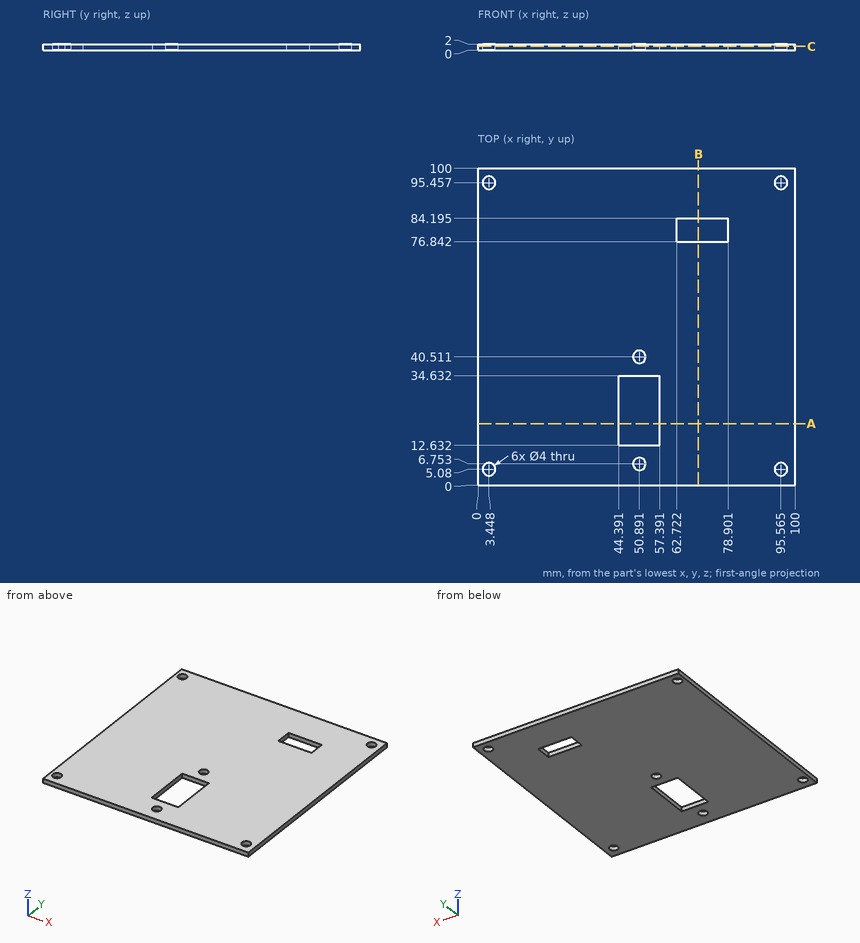
Input: dimensioned drawing with shaded views. Units: mm. Origin: part minimum x, y, z. Give positions to 0.01 mm unless a question says otherwise; leave off trailing zeros. Loops run counter-clockwise (first coordinate to the right, second up) from the corner with the lowest first, then second, coordinate; pieces in that order, holes last. Notation, with made-up numbers: M 20,-33.5 L 55,-33.5 A25 ccw 55,-4.5 Z; hole C -38,-28 d5. An arc over 180 degrees is marked long. Put each result on its own line as item: value. Start each with the question number.
1) Contact query for a flat-ended pin moving along its axis: pin 1 (6 mm diameter, centred on x = 12, y = 49.5, fed in from -Z). Output: stop coordinate, or through.
2) Cut plane B-B (x = 69.5). Output: boundary loops of the cut face in (y, z) (1 decimal), then the cut area to 3 significant figures.
3) Cut plane A-A (y = 19.5). Output: boundary loops of the cut face in (x, z).
4) Cut plane C-C (z = 1.25). Give the number of separate pieces and of enclosed holes in the cut face, then the cut area to 3 significant figures.
5) Ray query, line 1 along Y through (x, z) = (55.5, 1.75); line 2 along Y through (x, z) = (67, 0.8) (1 decimal); line 3 along X through (y, z) = (27, 0.1). Return the intervals inside material, ascending.
Verdict:
1. pin 1: z = 0
2. outline: M 0,0 L 76.8,0 L 76.8,2 L 0,2 Z; M 84.2,0 L 100,0 L 100,2 L 84.2,2 Z
2. area: 185 mm2
3. outline: M 0,0 L 44.39,0 L 44.39,2 L 0,2 Z; M 57.39,0 L 100,0 L 100,2 L 57.39,2 Z
4. separate pieces: 1
4. enclosed holes: 8
4. area: 9,520 mm2
5. line 1: 0 to 12.63, 34.63 to 100
5. line 2: 0 to 76.8, 84.2 to 100
5. line 3: 0 to 44.39, 57.39 to 100
